Design review of the part shown in the three views and the two pictorial views. Dimensions are in mm from the part's minimum x, y and z. Give positions to 0.01 mm unless a question says otherwise; leave off trailing zeros. Loops run counter-clockwise (first coordinate to the right, second up) from the corner with the lowest first, then second, coordinate; pieces in that order, holes last. Notation, with made-up numbers: (53, -17.75) - (59, -17.75) arc R17 ccw to (59, 6.25) - close; hole circle Ø6 at (58, -10). An arc over 180 degrees is marked (long way). Use CSV: the item, a comma, the result in double quotes. Start each with the question number.
1. Take a section at D-D on y = 6. Give the boundary of the cut face in (x, z), plus the area to 3 significant figures.
2. Take a section at C-C on z = 66. Give the boundary of the cut face in (x, y), plus the area to 3 significant figures.
3. Wall thickness on line 1 (Z direction, x = 63.5, y = 81.5); line 2 (Z direction, x = 78, y = 70); line 3 (X direction, y = 7, z = 30.5): over which ranges is each line inside the solid? List them lowest first.
4. Take a section at A-A on y = 25.5. Give the boundary of the cut face in (x, z).
5. For pin 1 (19 mm diameter, centred on y = 33.95, z = 62.854, fed in from -X); pin 2 (1 mm diameter, centred on y = 11, z = 50, fed in from +X); pin 3 (2 mm diameter, centred on y = 17.5, z = 101, fed in from +X); pin 4 (5 mm diameter, centred on x = 23, z = 21, fed in from +Y), all flat-tipped, find the tip position at first contact; note any pin that passes through.
6. Take a section at B-B on x = 82.5. Give the boundary of the cut face in (y, z).
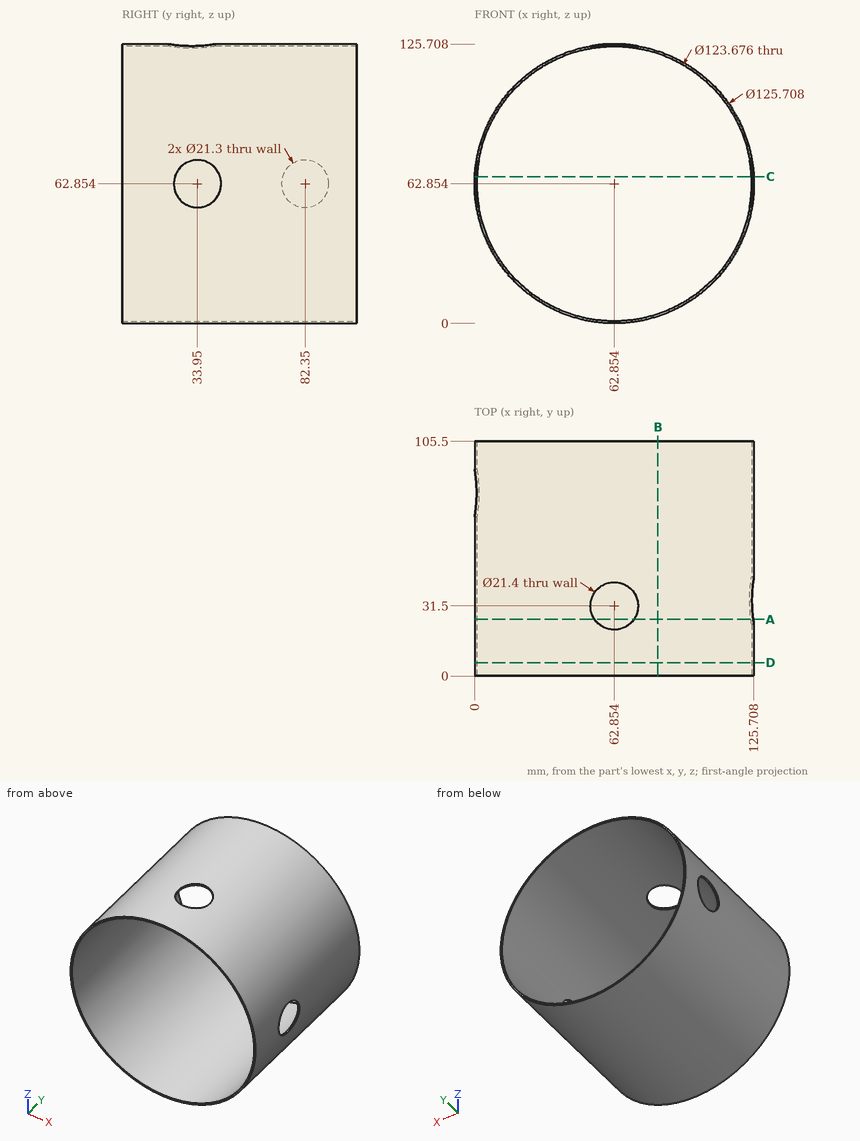
Check result:
1,outline,"circle Ø125.71 at (62.85, 62.85); hole circle Ø123.68 at (62.85, 62.85)"
1,area,"398 mm²"
2,outline,"(0.08, 0) - (1.1, 0) - (1.1, 72.18) - (0.08, 72.18) - close; (0.08, 92.52) - (1.1, 92.52) - (1.1, 105.5) - (0.08, 105.5) - close; (124.61, 0) - (125.63, 0) - (125.63, 23.78) - (124.61, 23.78) - close; (124.61, 44.12) - (125.63, 44.12) - (125.63, 105.5) - (124.61, 105.5) - close"
2,area,"173 mm²"
3,line 1,"z = 0 to 1.02, 124.69 to 125.7"
3,line 2,"z = 1.85 to 2.9, 122.81 to 123.86"
3,line 3,"x = 8.97 to 10.16, 115.55 to 116.74"
4,outline,"(53.99, 124.05) - (53.99, 125.08) arc R62.85 ccw (long way) to (125.37, 56.37) - (124.35, 56.37) arc R61.84 cw (long way) to start; (71.71, 124.05) arc R61.84 cw to (124.35, 69.34) - (125.37, 69.34) arc R62.85 ccw to (71.71, 125.08) - close"
5,pin 1,"stops at x = 0"
5,pin 2,"stops at x = 124.48"
5,pin 3,"stops at x = 113.56"
5,pin 4,"passes through"
6,outline,"(0, 3.15) - (105.5, 3.15) - (105.5, 4.22) - (0, 4.22) - close; (0, 121.49) - (105.5, 121.49) - (105.5, 122.56) - (0, 122.56) - close"
